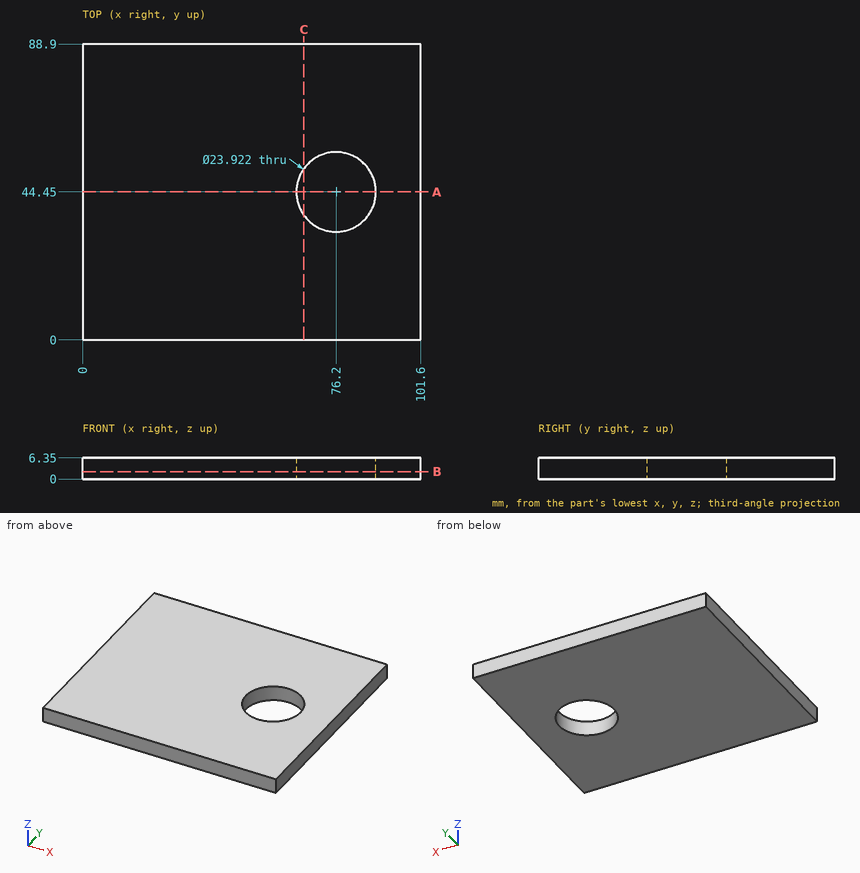
Check sheet for the drawn part. Datum: minimum x, y, z corner. Units: mm. Give positions to 0.01 mm unless a question says otherwise; leave off trailing zeros. Write each loop counter-clockwise with the first axis right and the second up, starting at its lowest first coordinate (ties: lowest second). Pieces come first, ordered by that corner, then holes. Notation, with made-up numbers: (17.25, -16) -> (50.25, -16) arc R11 cw to (50.25, -8) -> close; hole circle Ø3 at (30.5, -13). An arc over 180 degrees is marked (long way). Use one line per item in the form item = value. Start each with the question number.
1. Section check B-B (z = 2.25). Record the cut outline in (x, y).
2. Go/stop test with flat-tipped pins: P1, Ø1.5, axis at x = 39.5, y = 30, coming from the -Z side; P2, Ø19, axis at x = 76.2, y = 44.45, coming from the -Z side. Record where each tip stops, or that it passes through.
3. Section check C-C (x = 66.5). Record the cut outline in (y, z).
4. Section check A-A (y = 44.45). Record the cut outline in (x, z).
5. Thickness scan on line 1 along Y through (x, z) = (76.2, 2.75); line 2 along Y through (x, z) = (80, 3); line 3 along X through (y, z) = (47.5, 6.25) (1 decimal). Record the ranges inside material, lowest first. Write a range as from..to.
Conclusion:
q1.outline = (0, 0) -> (101.6, 0) -> (101.6, 88.9) -> (0, 88.9) -> close; hole circle Ø23.92 at (76.2, 44.45)
q2.P1 = 0
q2.P2 = through
q3.outline = (0, 0) -> (37.45, 0) -> (37.45, 6.35) -> (0, 6.35) -> close; (51.45, 0) -> (88.9, 0) -> (88.9, 6.35) -> (51.45, 6.35) -> close
q4.outline = (0, 0) -> (64.24, 0) -> (64.24, 6.35) -> (0, 6.35) -> close; (88.16, 0) -> (101.6, 0) -> (101.6, 6.35) -> (88.16, 6.35) -> close
q5.line_1 = 0..32.49, 56.41..88.9
q5.line_2 = 0..33.11, 55.79..88.9
q5.line_3 = 0..64.6, 87.8..101.6
